```python
from build123d import *

# Parameters (mm, degrees)
BOSS_EXTRUDE1_DEPTH = 1
SKETCH3_R           = 2.5
BOSS_EXTRUDE2_DEPTH = 5.4
FILLET1_R           = 0.3
SKETCH4_W           = 0.65
SKETCH4_H           = 2.2
BOSS_EXTRUDE3_DEPTH = 0.3
BOSS_EXTRUDE4_DEPTH = 0.01


with BuildPart() as part:
    # Sketch2 → Boss-Extrude1 (new body)
    with BuildSketch(Plane(origin=(0, 0, 0), x_dir=(1, 0, 0), z_dir=(0, 1, 0))):
        Polygon((2.65, -2.65), (-2.65, -2.65), (-2.65, 1.85), (-1.85, 2.65), (1.85, 2.65), (2.65, 1.85), align=None)
    extrude(amount=BOSS_EXTRUDE1_DEPTH)

    # Sketch3 → Boss-Extrude2 (add)
    with BuildSketch(Plane(origin=(0, 0, 0), x_dir=(1, 0, 0), z_dir=(0, 1, 0))):
        Circle(SKETCH3_R)
    extrude(amount=BOSS_EXTRUDE2_DEPTH)

    # Fillet1
    fillet1_edges = [part.edges().sort_by_distance(p)[0] for p in [
        (-2.5, 5.4, 0),
    ]]
    fillet(fillet1_edges, radius=FILLET1_R)

    # Sketch4 → Boss-Extrude3 (add)
    with BuildSketch(Plane(origin=(0, 0, 0), x_dir=(1, 0, 0), z_dir=(0, 1, 0))):
        with Locations((0, 1.85)):
            Rectangle(SKETCH4_W, SKETCH4_H)
        with Locations((0, -1.85)):
            Rectangle(SKETCH4_W, SKETCH4_H)
    extrude(amount=BOSS_EXTRUDE3_DEPTH)

    # Sketch5 → Boss-Extrude4 (add)
    with BuildSketch(Plane(origin=(0, 5.4, 0), x_dir=(1, 0, 0), z_dir=(0, 1, 0))):
        with BuildLine():
            Line((-1.984482533, -0.949646816), (1.984482533, -0.949646816))
            ThreePointArc((1.984482533, -0.949646816), (0, -2.2), (-1.984482533, -0.949646816))
        make_face()
    extrude(amount=BOSS_EXTRUDE4_DEPTH)


solid = part.part
```
Geometry: final body of the model. Coordinates: model frame, mm. A direction names the side the tool comes from. Round coordinates to 2 decimals unless told otherwise and drop trailing zeros. Write each loop counter-clockwise with the first axis right and the second up, starting at its lowest first coordinate (ties: lowest second). Pieces come first, ordered by that corner, then holes. Notation, with made-up numbers: M -38,79.25 L -30,79.25 A29 cw -30,106.25 Z; hole C 9,-0.75 d2. An arc over 180 degrees is marked long. Answer in a Markdown table with one row per item. Add a question column.
(1) Cut plane A-A, the plane z = 0. Return the cut outline in (x, y).
(2) Reachability of faces 1 (the face through (0, 0, 0)), 2 (the face through (0, 5.4, 0)), 3 (the face through (-0.54, 3.02, 2.44)) from +Z, -Z, +X, -X, +Y, -Y: full face, straight path, thin tool, end or side. Return the list, or none.
(3) Ray query, L1, parallel to Y at x = 0.7, z = -0.65; L2, parallel to Z at x = -1.55, y = 0.5; L3, parallel to Y at x = 1.6, z = 2. Return the intervals inside material, ascending.
(4) Contact query for flat-ended pins moving along their axis: pin 1 (1.6 mm diameter, centred on x = 0, z = -0.5, fed in from +Y); pin 2 (1.5 mm diameter, centred on x = 1, y = 1.5, fed in from -Z). Output: stop coordinate, or through.
(5) Cut plane D-D, the plane y = 2.05. Return the cut outline in (x, z).
(6) Cut plane B-B, the plane y = 0.85. Return the cut outline in (x, z).
Established:
| question | item | result |
|---|---|---|
| 1 | outline | M -2.65,0 L 2.65,0 L 2.65,1 L 2.5,1 L 2.5,5.1 A0.3 ccw 2.2,5.4 L -2.2,5.4 A0.3 ccw -2.5,5.1 L -2.5,1 L -2.65,1 Z |
| 2 | face 1 | +Z, -Z, +X, -X, -Y |
| 2 | face 2 | -Z, +X, -X, +Y |
| 2 | face 3 | +Y |
| 3 | L1 | 0 to 5.4 |
| 3 | L2 | -2.65 to 2.65 |
| 3 | L3 | 0 to 1 |
| 4 | pin 1 | y = 5.4 |
| 4 | pin 2 | z = -2.65 |
| 5 | outline | C 0,0 d5 |
| 6 | outline | M -2.65,-1.85 L -1.85,-2.65 L 1.85,-2.65 L 2.65,-1.85 L 2.65,2.65 L -2.65,2.65 Z |
